Geometry check sheet. Reference: the model listing, model coordinates, mm. A direction names the side the tool comes from. Coordinates: 2 decimals unless noted, no trailing zeros. Order: outer loops, then holes, each group sorted by start corner. A loop starts at its lowest first (then second) coordinate and runs counter-clockwise, first axis right, second up. Notation, with made-up numbers: (47, 69.5) - (55, 69.5) arc R19 cw to (55, 85.5) - close; hole circle Ø3 at (79, 41.5). An arc over 180 degrees is marked (long way). Put each result on its own line as item: value.
from build123d import *

# Parameters (mm, degrees)
CROQUIS1_R              = 2
SALIENTE_EXTRUIR1_DEPTH = 5
CROQUIS2_R              = 2
SALIENTE_EXTRUIR2_DEPTH = 5


with BuildPart() as part:
    # Croquis1 → Saliente-Extruir1 (new body)
    with BuildSketch(Plane.XY):
        with BuildLine():
            Line((-25.953664325, 5.804713338), (22.678050908, 5.804713338))
            ThreePointArc((22.678050908, 5.804713338), (27.678050908, 0.804713338), (22.678050908, -4.195286662))
            Line((22.678050908, -4.195286662), (-23.047151147, -4.195286662))
            ThreePointArc((-23.047151147, -4.195286662), (-41.661617991, 4.287687085), (-51.741257509, 22.088251307))
            ThreePointArc((-51.741257509, 22.088251307), (-48.695784379, 32.499543684), (-42.578743977, 23.541210565))
            ThreePointArc((-42.578743977, 23.541210565), (-36.695300038, 12.396079877), (-25.953664325, 5.804713338))
        make_face()
        with Locations((-17.321949092, 0.804713338)):
            Circle(CROQUIS1_R, mode=Mode.SUBTRACT)
    extrude(amount=SALIENTE_EXTRUIR1_DEPTH)

    # Croquis2 → Saliente-Extruir2 (add)
    with BuildSketch(Plane.XY.offset(5)):
        with Locations((22.678050908, 0.804713338)):
            Circle(CROQUIS2_R)
    extrude(amount=SALIENTE_EXTRUIR2_DEPTH)


solid = part.part
Q1. Section check D-D on z = 8.25. Record the boundary of the cut face in (x, y), then the cut area to 3 significant figures.
Answer block:
outline: circle Ø4 at (22.68, 0.8)
area: 12.6 mm^2
Q2. Thickness scan on L1, parallel to Y at x = 15.5, z = 3; L2, parallel to Z at x = 3.5, y = 4.5; L3, parallel to X at y = 0, z = 9.25. Record the ranges inside material, lowest first. Write a range as [from, to].
Answer block:
L1: y = [-4.2, 5.8]
L2: z = [0, 5]
L3: x = [20.85, 24.51]
Q3. Section check A-A on z = 2.25. Record the boundary of the cut face in (x, y), then the cut area to 3 significant figures.
Answer block:
outline: (-51.74, 22.09) arc R33.12 ccw to (-23.05, -4.2) - (22.68, -4.2) arc R5 ccw to (22.68, 5.8) - (-25.95, 5.8) arc R23.85 cw to (-42.58, 23.54) arc R6 ccw (long way) to start; hole circle Ø4 at (-17.32, 0.8)
area: 909 mm^2
Q4. Section check B-B on y = 4. Record the boundary of the cut face in (x, z), then the cut area to 3 significant figures.
Answer block:
outline: (-41.34, 0) - (26.52, 0) - (26.52, 5) - (-41.34, 5) - close
area: 339 mm^2
Q5. Draft check along X on faces 3 (the cylindrical face through (-16.247, 2.491, 2.465)), 4 (the flat face through (0, -4.195, 2)), 5 (the cylindrical face through (20.68, 0.89, 7.46)), 6 (the cylindrical face through (27.677, 0.915, 2.465)). Enter one of: pulls with the +X half, pulls with the -X half, needs draft (parallel to the pull), parting line crosses it, or undercut.
Answer block:
face 3: undercut
face 4: needs draft
face 5: parting line crosses it
face 6: pulls with the +X half
Q6. Section check C-C on x = 6. Record the boundary of the cut face in (y, z), then the cut area to 3 significant figures.
Answer block:
outline: (-4.2, 0) - (5.8, 0) - (5.8, 5) - (-4.2, 5) - close
area: 50.0 mm^2
Q7. Depth check by flat-ended pin: pin 1 Ø18.5 at (x, y) = (-6, 7.5) entering from +Z; pin 2 Ø6.5 at (x, y) = (-17.32, 0.8) entering from -Z; pin 3 Ø3 at (y, z) = (15.5, 3) entering from -X; pin 4 Ø1.5 at (x, z) = (3.5, 2) entering from +Y. Enter the tip coordinate at first touch or a pass-through.
Answer block:
pin 1: stops at z = 5
pin 2: stops at z = 0
pin 3: stops at x = -50.27
pin 4: stops at y = 5.8
Q8. Access from +Z, -Z, +X, -X, +Y, -Y to the whole of each face (thin tool, end or side, straight path). Record for faces 1 (the flat face through (-2, 5.805, 2)), 2 (the flat face through (23, 1, 10)).
Answer block:
face 1: +Z, -Z, +X, +Y
face 2: +Z, +X, -X, +Y, -Y
